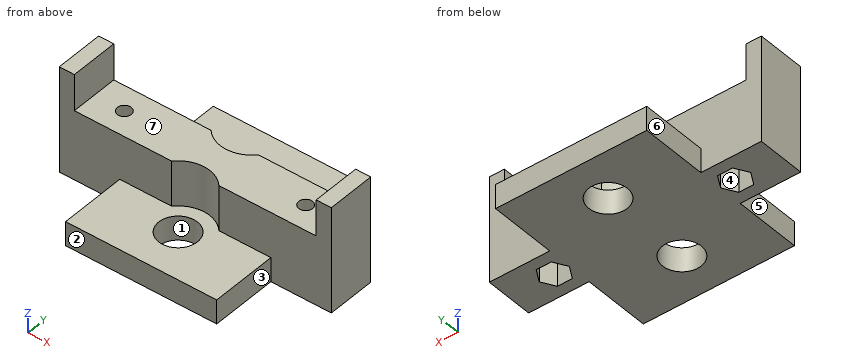
from build123d import *

# Parameters (mm, degrees)
SKETCH_1_W           = 25
SKETCH_1_H           = 30
SKETCH_1_R           = 3.2
EXTRUDE_1_DEPTH      = 4
SKETCH_2_W           = 40
SKETCH_2_H           = 8
SKETCH_2_R           = 1.15
EXTRUDE_2_DEPTH      = 7.5
EXTRUDE_2_DEPTH_BACK = 4
CUT_EXTRUDE_2_DEPTH  = 9.5
SKETCH_5_R           = 5.25
CUT_EXTRUDE_3_DEPTH  = 7.5
SKETCH_6_W           = 2.5
SKETCH_6_H           = 8
EXTRUDE_3_DEPTH      = 17.5


with BuildPart() as part:
    # 스케치1 → 보스-돌출1 (new body)
    with BuildSketch(Plane.XY):
        Rectangle(SKETCH_1_W, SKETCH_1_H)
        with Locations((0, 7.5)):
            Circle(SKETCH_1_R, mode=Mode.SUBTRACT)
        with Locations((0, -7.5)):
            Circle(SKETCH_1_R, mode=Mode.SUBTRACT)
    extrude(amount=EXTRUDE_1_DEPTH)

    # 스케치2 → 보스-돌출2 (add, two sides)
    with BuildSketch(Plane.XY.offset(4)) as extrude_2_sk:
        Rectangle(SKETCH_2_W, SKETCH_2_H)
        with Locations((15, 0)):
            Circle(SKETCH_2_R, mode=Mode.SUBTRACT)
        with Locations((-15, 0)):
            Circle(SKETCH_2_R, mode=Mode.SUBTRACT)
    extrude(amount=EXTRUDE_2_DEPTH)
    extrude(extrude_2_sk.sketch, amount=-EXTRUDE_2_DEPTH_BACK)

    # 스케치4 → 컷-돌출2 (cut)
    with BuildSketch(Plane(origin=(0, 0, 0), x_dir=(-1, 0, 0), z_dir=(0, 0, -1))):
        Polygon((17.482606158, 0), (16.241303079, 2.15), (13.758696921, 2.15), (12.517393842, 0), (13.758696921, -2.15), (16.241303079, -2.15), align=None)
        Polygon((-12.517393842, 0), (-13.758696921, 2.15), (-16.241303079, 2.15), (-17.482606158, 0), (-16.241303079, -2.15), (-13.758696921, -2.15), align=None)
    extrude(amount=-CUT_EXTRUDE_2_DEPTH, mode=Mode.SUBTRACT)

    # 스케치5 → 컷-돌출3 (cut)
    with BuildSketch(Plane.XY.offset(4)):
        with Locations((0, 7.5)):
            Circle(SKETCH_5_R)
        with Locations((0, -7.5)):
            Circle(SKETCH_5_R)
    extrude(amount=CUT_EXTRUDE_3_DEPTH, mode=Mode.SUBTRACT)

    # 스케치6 → 보스-돌출3 (add)
    with BuildSketch(Plane(origin=(0, 0, 0), x_dir=(-1, 0, 0), z_dir=(0, 0, -1))):
        with Locations((21.25, 0)):
            Rectangle(SKETCH_6_W, SKETCH_6_H)
        with Locations((-21.25, 0)):
            Rectangle(SKETCH_6_W, SKETCH_6_H)
    extrude(amount=-EXTRUDE_3_DEPTH)


solid = part.part
Geometry: final body of the model. Coordinates: model frame, mm. Face numbers are marked on the shaded views. A direction names the side the tool comes from. Give positions to 0.01 mm unless a question says otherwise; leave off trailing zeros. Order: outer loops, then holes, each group sorted by start corner. A loop starts at its lowest first (then second) coordinate and runs counter-clockwise, first axis right, second up. Notation, with made-up numbers: (-35, 83) -> (-29, 83) arc R23 cw to (-29, 92) -> close; hole circle Ø4 at (30.25, 53). An arc over 180 degrees is marked (long way). Put each result on its own line as item: value.
Q1. Section A-A, the plane z = 15.75. Return loops of the section in (x, y), then the cut area to 3 significant figures.
Here are the results:
outline: (-22.5, -4) -> (-20, -4) -> (-20, 4) -> (-22.5, 4) -> close; (20, -4) -> (22.5, -4) -> (22.5, 4) -> (20, 4) -> close
area: 40.0 mm^2
Q2. Reachability of the marked faces 4, 5, 6 and 7 from +Z, -Z, +X, -X, +Y, -Y: full face, straight path, thin tool, end or side. Return the list, or none.
Here are the results:
face 4: -Z
face 5: +Z, -Z, -X, -Y
face 6: +Z, -Z, -X, +Y
face 7: +Z, +Y, -Y
Q3. Material intervals for L1, parallel to X at y = 0, z = 9.9; L2, parallel to Y at x = 0, z = 1.6; L3, parallel to Y at x = 15, z = 10, sorted ascending.
Here are the results:
L1: x = -22.5 to -16.15, -13.85 to 13.85, 16.15 to 22.5
L2: y = -15 to -10.7, -4.3 to 4.3, 10.7 to 15
L3: y = -4 to -1.15, 1.15 to 4
Q4. Pin query (flat end, axial travel): pin 1 (9 mm diameter, centred on x = -1, y = -0.5, fed in from +Z); pin 2 (1.2 mm diameter, centred on y = -8, z = 1.5, fed in from +X); pin 3 (8 mm diameter, centred on x = -11, z = 9, fed in from -Y). Return the tip coordinate at first contact, or that it passes through.
Here are the results:
pin 1: stops at z = 11.5
pin 2: stops at x = 12.5
pin 3: stops at y = -4
Q5. Section D-D, the plane z = 3.25. Return loops of the section in (x, y).
Here are the results:
outline: (-22.5, -4) -> (-12.5, -4) -> (-12.5, -15) -> (12.5, -15) -> (12.5, -4) -> (22.5, -4) -> (22.5, 4) -> (12.5, 4) -> (12.5, 15) -> (-12.5, 15) -> (-12.5, 4) -> (-22.5, 4) -> close; hole (-17.48, 0) -> (-16.24, -2.15) -> (-13.76, -2.15) -> (-12.52, 0) -> (-13.76, 2.15) -> (-16.24, 2.15) -> close; hole circle Ø6.4 at (0, -7.5); hole circle Ø6.4 at (0, 7.5); hole (12.52, 0) -> (13.76, -2.15) -> (16.24, -2.15) -> (17.48, 0) -> (16.24, 2.15) -> (13.76, 2.15) -> close
Q6. Section B-B, the plane y = 7.5. Return loops of the section in (x, z).
Here are the results:
outline: (-12.5, 0) -> (-3.2, 0) -> (-3.2, 4) -> (-12.5, 4) -> close; (3.2, 0) -> (12.5, 0) -> (12.5, 4) -> (3.2, 4) -> close
Q7. Section C-C, the plane x = 15. Return loops of the section in (y, z), then the cut area to 4 significant figures.
Here are the results:
outline: (-4, 0) -> (-2.15, 0) -> (-2.15, 9.5) -> (-1.15, 9.5) -> (-1.15, 11.5) -> (-4, 11.5) -> close; (1.15, 9.5) -> (2.15, 9.5) -> (2.15, 0) -> (4, 0) -> (4, 11.5) -> (1.15, 11.5) -> close
area: 46.55 mm^2
Q8. Draft query along Y for the marked faces 1, 2 and 3. Return one class per face: released by +Y, released by -Y, zero draft, split by the parting line, or undercut.
Here are the results:
face 1: undercut
face 2: released by -Y
face 3: zero draft
